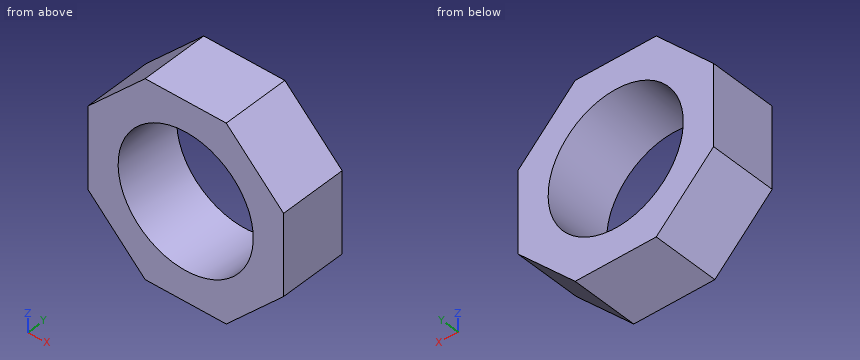
from build123d import *

# Parameters (mm, degrees)
ESBO_O1_R                = 5
RESSALTO_EXTRUS_O1_DEPTH = 5


with BuildPart() as part:
    # Esboço1 → Ressalto-extrusão1 (new body)
    with BuildSketch(Plane(origin=(0, 0, 0), x_dir=(1, 0, 0), z_dir=(0, 1, 0))):
        Polygon((-3, 7.242640687), (3, 7.242640687), (7.242640687, 3), (7.242640687, -3), (3, -7.242640687), (-3, -7.242640687), (-7.242640687, -3), (-7.242640687, 3), align=None)
        with Locations(Location((0, 0, 0), (0, 0, 270))):
            Circle(ESBO_O1_R, mode=Mode.SUBTRACT)
    extrude(amount=RESSALTO_EXTRUS_O1_DEPTH)


solid = part.part
The model under review builds one solid part; all positions refer to its coordinate system, in mm. Coordinates: 2 decimals unless noted, no trailing zeros. Write each loop counter-clockwise with the first axis right and the second up, starting at its lowest first coordinate (ties: lowest second). Pieces come first, ordered by that corner, then holes. Notation, with made-up numbers: (-39, 69) - (12, 69) arc R25 cw to (12, 108) - close; hole circle Ø11 at (75.25, -15). An arc over 180 degrees is marked (long way). Answer as CSV lines item,"result".
(1) We need section D-D (z = -5.25). Give the boundary of the cut face in (x, y), plus the area to 3 significant figures.
Data:
outline,"(-4.99, 0) - (4.99, 0) - (4.99, 5) - (-4.99, 5) - close"
area,"49.9 mm2"
(2) Clearance check with a flat-ended pin moving along its axis: pin 1 Ø1 at (x, y) = (4, 2) entering from +Z. State where the tip first meets the part, or that it passes through.
Data:
pin 1,"stops at z = 6.74"
(3) We need section B-B (x = 0). Give the boundary of the cut face in (y, z), plus the area to 3 significant figures.
Data:
outline,"(0, -7.24) - (5, -7.24) - (5, -5) - (0, -5) - close; (0, 5) - (5, 5) - (5, 7.24) - (0, 7.24) - close"
area,"22.4 mm2"
(4) We need section A-A (z = 0). Give the boundary of the cut face in (x, y), plus the area to 3 significant figures.
Data:
outline,"(-7.24, 0) - (-5, 0) - (-5, 5) - (-7.24, 5) - close; (5, 0) - (7.24, 0) - (7.24, 5) - (5, 5) - close"
area,"22.4 mm2"
(5) We need section C-C (y = 2.55). Give the boundary of the cut face in (x, z), plus the area to 3 significant figures.
Data:
outline,"(-7.24, -3) - (-3, -7.24) - (3, -7.24) - (7.24, -3) - (7.24, 3) - (3, 7.24) - (-3, 7.24) - (-7.24, 3) - close; hole circle Ø10 at (0, 0)"
area,"95.3 mm2"
(6) For line 1 along X through (y, z) = (1.75, 0); line 2 along X through (y, z) = (1.55, -1.75); line 3 along Z through (x, y) = (-4, 2.05), list the stretches that pass through material, from the lowest coordinate up. Write a range as [from, to].
Data:
line 1,"x = [-7.24, -5], [5, 7.24]"
line 2,"x = [-7.24, -4.68], [4.68, 7.24]"
line 3,"z = [-6.24, -3], [3, 6.24]"
